from build123d import *

# Parameters (mm, degrees)
SKETCH1_R           = 1.5
BOSS_EXTRUDE1_DEPTH = 3
FILLET1_R           = 10


with BuildPart() as part:
    # Sketch1 → Boss-Extrude1 (new body)
    with BuildSketch(Plane.XY):
        with BuildLine():
            Line((0, 10), (-4.960783708, 5.625))
            ThreePointArc((-4.960783708, 5.625), (-3.085783708, -6.835783708), (7.5, 0))
            Line((7.5, 0), (142.5, 0))
            ThreePointArc((142.5, 0), (153.085783708, -6.835783708), (154.960783708, 5.625))
            Line((154.960783708, 5.625), (150, 10))
            Line((150, 10), (0, 10))
        make_face()
        Circle(SKETCH1_R, mode=Mode.SUBTRACT)
        with Locations((150, 0)):
            Circle(SKETCH1_R, mode=Mode.SUBTRACT)
    extrude(amount=BOSS_EXTRUDE1_DEPTH)

    # Fillet1
    fillet1_edges = [part.edges().sort_by_distance(p)[0] for p in [
        (7.5, 0, 1.5),
        (0, 10, 1.5),
        (150, 10, 1.5),
        (142.5, 0, 1.5),
    ]]
    fillet(fillet1_edges, radius=FILLET1_R)


solid = part.part
Geometry check sheet. Reference: the model listing, model coordinates, mm. A direction names the side the tool comes from. Coordinates: 2 decimals unless noted, no trailing zeros. Order: outer loops, then holes, each group sorted by start corner. A loop starts at its lowest first (then second) coordinate and runs counter-clockwise, first axis right, second up. Notation, with made-up numbers: (23.5, 82.25) - (45.5, 82.25) arc R29 cw to (45.5, 115.25) - close; hole circle Ø3 at (0, -0.5). An arc over 180 degrees is marked (long way). Answer in a Markdown table with one row per item. Add a question column.
1) Release check for a two-part mould opening along X. For faces 1 (the cylindrical face through (0.197, 9.336, 1.521)), 2 (the flat face through (76, 10, 1)), 3 (the cylindrical face through (140, -1, 2)), 4 (the cylindrical face through (148.5, 0.07, 1.48)) record: +X half, -X half, draft (parallel to the pull), parting line (faces both ways), or undercut.
2) Cross-section at B-B, the plane x = 150. Record the cut outline in (y, z).
3) Material ranges on line 1 along Y through (x, z) = (150, 1); line 2 along X through (y, z) = (-4, 0.1); line 3 along Y through (x, z) = (25, 0.1), recorded low to high. Write a range as [from, to].
4) Set-up check for faces 5 (the cylindrical face through (149.71, 9.37, 1.52)), 6 (the flat face through (74, 0, 1)): record each of +Z, -Z, +X, -X, +Y, -Y from which the full face is reachable in a straight line by a thin tool's end or side.
5) Cross-section at A-A, the plane z = 2.25. Record the cut outline in (x, y) (3 decimals).
6) Cross-section at C-C, the plane x = 110. Record the cut outline in (y, z).
7) Gauge pin test, flat ends, axial feed: P1, Ø4, axis at x = 0, y = 0, coming from the +Z side; P2, Ø1.5, axis at y = 4, z = 0.5, coming from the +X side; P3, Ø1.5, axis at x = 91.5, z = 1.5, coming from the -Y side. Record the tip position at first contact, or that the pin passes through.
Check result:
| question | item | result |
|---|---|---|
| 1 | face 1 | -X half |
| 1 | face 2 | draft |
| 1 | face 3 | undercut |
| 1 | face 4 | undercut |
| 2 | outline | (-7.5, 0) - (-1.5, 0) - (-1.5, 3) - (-7.5, 3) - close; (1.5, 0) - (9.26, 0) - (9.26, 3) - (1.5, 3) - close |
| 3 | line 1 | y = [-7.5, -1.5], [1.5, 9.26] |
| 3 | line 2 | x = [-6.34, 6.36], [143.64, 156.34] |
| 3 | line 3 | y = [0, 10] |
| 4 | face 5 | +Z, -Z, +X, +Y |
| 4 | face 6 | +Z, -Z, -Y |
| 5 | outline | (-4.961, 5.625) arc R7.5 ccw (long way) to (6.155, -4.286) arc R10 cw to (14.361, 0) - (135.639, 0) arc R10 cw to (143.845, -4.286) arc R7.5 ccw (long way) to (154.961, 5.625) - (152.835, 7.5) arc R10 ccw to (146.22, 10) - (3.78, 10) arc R10 ccw to (-2.835, 7.5) - close; hole circle Ø3 at (0, 0); hole circle Ø3 at (150, 0) |
| 6 | outline | (0, 0) - (10, 0) - (10, 3) - (0, 3) - close |
| 7 | P1 | stops at z = 3 |
| 7 | P2 | stops at x = 156.76 |
| 7 | P3 | stops at y = 0 |
